```python
from build123d import *

# Parameters (mm, degrees)
F0_R           = 1.5875
F0_W           = 50.8
F0_H           = 25.4
F1_DEPTH       = 9.525
F2_R           = 3.175
F4_D           = 4.7625
F4_CSINK_D     = 9.525
F4_CSINK_ANGLE = 90


with BuildPart() as f1:
    # F0 (on Front) → F1 (new body)
    with BuildSketch(Plane.XZ):
        with BuildLine():
            Line((0, 25.4), (0, 0))
            Line((0, 0), (206.375, 0))
            Line((206.375, 0), (206.375, 25.4))
            Line((206.375, 25.4), (204.7875, 25.4))
            ThreePointArc((204.7875, 25.4), (201.6125, 28.575), (204.7875, 31.75))
            Line((204.7875, 31.75), (206.375, 31.75))
            Line((206.375, 31.75), (214.3125, 31.75))
            Line((214.3125, 31.75), (214.3125, 50.8))
            Line((214.3125, 50.8), (206.375, 50.8))
            Line((206.375, 50.8), (0, 50.8))
            Line((0, 50.8), (-7.9375, 50.8))
            Line((-7.9375, 50.8), (-7.9375, 31.75))
            Line((-7.9375, 31.75), (0, 31.75))
            Line((0, 31.75), (1.5875, 31.75))
            ThreePointArc((1.5875, 31.75), (3.832564, 30.820064), (4.7625, 28.575))
            ThreePointArc((4.7625, 28.575), (3.832564, 26.329936), (1.5875, 25.4))
            Line((1.5875, 25.4), (0, 25.4))
        make_face()
        with Locations((11.1125, 15.875)):
            Circle(F0_R, mode=Mode.SUBTRACT)
        with Locations((47.625, 15.875)):
            Circle(F0_R, mode=Mode.SUBTRACT)
        with Locations((103.1748, 25.4)):
            Rectangle(F0_W, F0_H, mode=Mode.SUBTRACT)
        with Locations((158.7246, 15.875)):
            Circle(F0_R, mode=Mode.SUBTRACT)
        with Locations((195.2498, 15.875)):
            Circle(F0_R, mode=Mode.SUBTRACT)
        with Locations((11.1125, 34.925)):
            Circle(F0_R, mode=Mode.SUBTRACT)
        with Locations((47.625, 34.925)):
            Circle(F0_R, mode=Mode.SUBTRACT)
        with Locations((158.7246, 34.925)):
            Circle(F0_R, mode=Mode.SUBTRACT)
        with Locations((195.2498, 34.925)):
            Circle(F0_R, mode=Mode.SUBTRACT)
    extrude(amount=F1_DEPTH)

    # F2
    f2_edges = [f1.edges().sort_by_distance(p)[0] for p in [
        (77.7748, -4.7625, 12.7),
        (128.5748, -4.7625, 12.7),
        (77.7748, -4.7625, 38.1),
        (128.5748, -4.7625, 38.1),
    ]]
    fillet(f2_edges, radius=F2_R)

    # F4 (through all)
    with Locations(Plane.XY.offset(50.8)):
        with Locations((-3.96875, -4.7625), (210.34375, -4.7625)):
            CounterSinkHole(F4_D / 2, F4_CSINK_D / 2, counter_sink_angle=F4_CSINK_ANGLE)


solid = f1.part
```
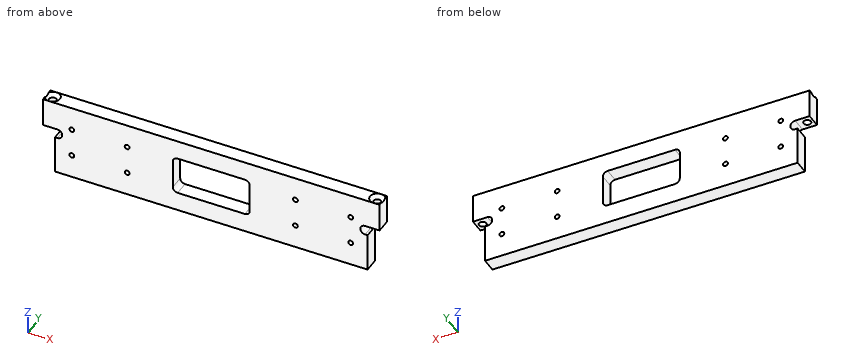
Geometry check sheet. Reference: the model listing, model coordinates, mm. Round coordinates to 2 decimals unless told otherwise and drop trailing zeros. Loops run counter-clockwise (first coordinate to the right, second up) from the corner with the lowest first, then second, coordinate; pieces in that order, holes last. Notation, with made-up numbers: (-23.5, 11) - (31.5, 11) arc R9 ccw to (31.5, 15) - close; hole circle Ø2 at (-34, 50.5). An arc over 180 degrees is marked (long way). Write each question's results on one line, items separated by ' | '. Start each with the question number.
Q1. Gauge pin test, flat ends, axial feed: P1, Ø2, axis at y = -4.5, z = 5.5, coming from the +X side (3 decimals); P2, Ø1.5, axis at y = -7, z = 24.5, coming from the -X side; P3, Ø3, axis at x = -4.5, y = -7, coming from the -Z side. Record the tip position at first contact, or that the pin passes through.
Q2. Cross-section at B-B on z = 22. Enter the section's corners in (x, y) (3 decimals), and give its area (3 significant figures).
Q3. Cross-section at A-A on x = 117. Enter the section's corners in (y, z) (3 decimals).
Q4. Thickness scan on line 1 (X direction, y = -1.5, z = 18.5) (3 decimals); line 2 (X direction, y = -3.75, z = 40); line 3 (X direction, y = -7.25, z = 33). Record the ranges inside material, lowest first. Write a range as [from, to].
Q5. Cross-section at C-C on z = 41. State how many separate pieces and enclosed holes the cut face has, and give its area (3 significant figures).
Answers below:
1) P1: stops at x = 206.375 | P2: stops at x = 0 | P3: stops at z = 31.75
2) outline: (0, -9.525) - (77.775, -9.525) - (77.775, 0) - (0, 0) - close; (128.575, -9.525) - (206.375, -9.525) - (206.375, 0) - (128.575, 0) - close | area: 1,480 mm²
3) outline: (-9.525, 0) - (0, 0) - (0, 12.7) - (-9.525, 12.7) - close; (-9.525, 38.1) - (0, 38.1) - (0, 50.8) - (-9.525, 50.8) - close
4) line 1: x = [0, 77.775], [128.575, 206.375] | line 2: x = [-7.94, -6.12], [-1.81, 208.19], [212.5, 214.31] | line 3: x = [-7.94, 77.77], [128.57, 214.31]
5) separate pieces: 1 | enclosed holes: 2 | area: 2,080 mm²
